Geometry check sheet. Reference: the model listing, model coordinates, mm. A direction names the side the tool comes from. Round coordinates to 2 decimals unless told otherwise and drop trailing zeros. Order: outer loops, then holes, each group sorted by start corner. A loop starts at its lowest first (then second) coordinate and runs counter-clockwise, first axis right, second up.
(1) Cross-section at B-B on x = 29. Enter the section's corners in (y, z).
(2) Set-up check for faces 1 (the face through (6.2, 3, -10)), 2 (the face through (8.6, 5.2, -14.2)), 3 (the face through (26.78, 3, -32)), 4 (the face through (3, 3, -24.66)), 5 (the face through (12, 3, -35)): record each of +Z, -Z, +X, -X, +Y, -Y from which the full face is reachable in a straight line by a thin tool's end or side.
(3) Gauge pin test, flat ends, axial feed: P1, Ø2, axis at x = 16, y = 2.5, coming from the -Z side; P2, Ø3, axis at x = 2, y = 3.5, coming from the +Z side; P3, Ø3, axis at y = 2, z = -33, coming from the -X side. Record the tip position at first contact, or that the pin passes through.
(4) Thickness scan on L1, parallel to X at y = 2, z = -32.5; L2, parallel to X at y = 3.5, z = -25; L3, parallel to Z at x = 30.5, y = 2.75. Record the ranges inside material, lowest first.
(5) Cross-section at C-C on z = -20. Enter the section's corners in (x, y).
(6) Cross-section at D-D on y = 2. Count the separate pieces of the cut face and the enclosed holes in it, and give its area (3 significant figures).
(7) Draft check along Z on faces 6 (the face through (3, 3, -4.11)), 7 (the face through (7.9, 5.71, -14.66)), 8 (the face through (0, 3, -6)). Enter one of: pulls with the +Z half, pulls with the -Z half, needs draft (parallel to the pull), parting line crosses it, or undercut.
(8) Cross-section at A-A on x = 5.5. Enter the section's corners in (y, z).
from build123d import *

# Parameters (mm, degrees)
SKETCH1_R           = 2.5
BOSS_EXTRUDE1_DEPTH = 6.2
CUT_EXTRUDE1_DEPTH  = 1


with BuildPart() as part:
    # Sketch1 → Boss-Extrude1 (new body)
    with BuildSketch(Plane(origin=(0, 0, 0), x_dir=(1, 0, 0), z_dir=(0, 1, 0))):
        Polygon((0, 24.66), (0, 20.55), (6.2, 20.55), (6.2, 16.44), (0, 16.44), (0, 12.33), (6.2, 12.33), (6.2, 8.22), (0, 8.22), (0, 4.11), (6.2, 4.11), (6.2, 0), (17, 0), (35, 0), (35, 18), (35, 28.8), (30.89, 28.8), (30.89, 35), (26.78, 35), (26.78, 28.8), (22.67, 28.8), (22.67, 35), (18.56, 35), (18.56, 28.8), (14.45, 28.8), (14.45, 35), (10.34, 35), (10.34, 28.8), (6.2, 28.8), (6.2, 24.66), align=None)
        with Locations((10.006, 25)):
            Circle(SKETCH1_R, mode=Mode.SUBTRACT)
        with Locations((30.02235364, 4.980572344)):
            Circle(SKETCH1_R, mode=Mode.SUBTRACT)
    extrude(amount=BOSS_EXTRUDE1_DEPTH)

    # Sketch2 → Cut-Extrude1 (cut)
    with BuildSketch(Plane(origin=(0, 6.2, 0), x_dir=(1, 0, 0), z_dir=(0, 1, 0))):
        with BuildLine():
            Line((9.367624272, 15.46006193), (9.367624272, 15.134420905))
            Line((9.367624272, 15.134420905), (8.28766634, 15.134420905))
            Line((8.28766634, 15.134420905), (8.116577598, 14.299329759))
            add(Edge.make_bspline(
                [(8.116577598, 14.299329759), (8.150192569, 14.308610077), (8.215316261, 14.326589225), (8.311436992, 14.346551603), (8.40268849, 14.358585256), (8.461902576, 14.360228373), (8.490555963, 14.361023469)],
                knots=[0, 0, 0, 0, 0.000104595, 0.000202637, 0.000294305, 0.000380252, 0.000380252, 0.000380252, 0.000380252], degree=3))
            add(Edge.make_bspline(
                [(8.490555963, 14.361023469), (8.526010498, 14.360256084), (8.595722973, 14.358747215), (8.697721161, 14.344258466), (8.795087428, 14.321452972), (8.88761815, 14.289593641), (8.975484506, 14.248854097), (9.05787808, 14.197963437), (9.136035615, 14.138515344), (9.208554968, 14.070166655), (9.274344876, 13.994944902), (9.332189738, 13.914065976), (9.381322945, 13.828315883), (9.420838773, 13.736875331), (9.452393133, 13.640755241), (9.4733953, 13.538944256), (9.487380458, 13.432402033), (9.488942908, 13.359554316), (9.489739657, 13.322406682)],
                knots=[0, 0, 0, 0, 0.000106308, 0.000209029, 0.000308378, 0.000405929, 0.000502102, 0.000598312, 0.00069588, 0.000796219, 0.000896736, 0.000995218, 0.001094066, 0.001192613, 0.001293582, 0.001396995, 0.001504047, 0.001615439, 0.001615439, 0.001615439, 0.001615439], degree=3))
            add(Edge.make_bspline(
                [(9.489739657, 13.322406682), (9.489136339, 13.296532954), (9.487937855, 13.245135158), (9.481843137, 13.168804347), (9.470108594, 13.094089491), (9.454353587, 13.020980679), (9.433904394, 12.94961632), (9.409149323, 12.879792148), (9.378854356, 12.811942755), (9.345624465, 12.745426146), (9.308208017, 12.681746072), (9.266680371, 12.622193063), (9.222805961, 12.56587375), (9.17559699, 12.51339215), (9.124614659, 12.465093126), (9.070476403, 12.420690042), (9.013614223, 12.379431978), (8.953148396, 12.342993687), (8.890426286, 12.309463005), (8.824542118, 12.281955225), (8.756995625, 12.257362103), (8.686814631, 12.237759175), (8.614158101, 12.222398929), (8.538906269, 12.211966241), (8.461453804, 12.204367616), (8.4089529, 12.203891949), (8.382432966, 12.203651674)],
                knots=[0, 0, 0, 0, 7.7636e-05, 0.000154223, 0.000229512, 0.000304362, 0.000378447, 0.000452077, 0.000526407, 0.000601214, 0.00067506, 0.000747747, 0.00081887, 0.000889121, 0.000959302, 0.001029336, 0.001099058, 0.00116985, 0.001240974, 0.00131221, 0.00138383, 0.001456517, 0.001530612, 0.001606437, 0.001684346, 0.001763871, 0.001763871, 0.001763871, 0.001763871], degree=3))
            add(Edge.make_bspline(
                [(8.382432966, 12.203651674), (8.350797102, 12.204278363), (8.288557277, 12.205511299), (8.197370763, 12.218409496), (8.109636799, 12.236882477), (8.026061636, 12.264673951), (7.945896275, 12.299496711), (7.870219953, 12.343507809), (7.797098999, 12.393381711), (7.729505937, 12.452237459), (7.666771462, 12.516568114), (7.610613415, 12.586379688), (7.560599385, 12.660519968), (7.517530286, 12.739349008), (7.480792795, 12.822659675), (7.451932056, 12.910764112), (7.428638119, 13.003201972), (7.418783445, 13.066841228), (7.413778118, 13.099164495)],
                knots=[0, 0, 0, 0, 9.4843e-05, 0.000186593, 0.000275792, 0.000363484, 0.000450342, 0.000537514, 0.000625728, 0.000715478, 0.000805885, 0.000894984, 0.00098389, 0.001073836, 0.001164117, 0.001256635, 0.001351658, 0.001449737, 0.001449737, 0.001449737, 0.001449737], degree=3))
            Line((7.413778118, 13.099164495), (7.698714016, 13.099164495))
            add(Edge.make_bspline(
                [(7.698714016, 13.099164495), (7.705724921, 13.068887284), (7.719200271, 13.010692804), (7.748778343, 12.928930802), (7.784942388, 12.856069792), (7.827944904, 12.791145956), (7.87924386, 12.73453208), (7.93778127, 12.684079459), (8.003410991, 12.638563449), (8.076339135, 12.600624224), (8.153276714, 12.56826757), (8.233801254, 12.546721389), (8.315720197, 12.531571293), (8.371127004, 12.530054768), (8.398969424, 12.5292927)],
                knots=[0, 0, 0, 0, 9.3172e-05, 0.000179081, 0.000260145, 0.000336703, 0.000411917, 0.000488562, 0.000568128, 0.000650923, 0.00073478, 0.000817953, 0.000900557, 0.000983994, 0.000983994, 0.000983994, 0.000983994], degree=3))
            add(Edge.make_bspline(
                [(8.398969424, 12.5292927), (8.426146013, 12.530037262), (8.479656939, 12.531503313), (8.558407269, 12.542787274), (8.634437519, 12.560165928), (8.706997478, 12.586173582), (8.777356875, 12.617782719), (8.843735938, 12.658345681), (8.908054976, 12.705027269), (8.968314783, 12.758509355), (9.023504855, 12.817446149), (9.072269336, 12.880472071), (9.112888394, 12.947706638), (9.147118621, 13.017985856), (9.173111256, 13.092079975), (9.191654146, 13.169641756), (9.202542635, 13.250862773), (9.204040492, 13.306261362), (9.204803759, 13.334491017)],
                knots=[0, 0, 0, 0, 8.15e-05, 0.000160473, 0.000238226, 0.000315066, 0.000391338, 0.000469218, 0.000547964, 0.000629516, 0.000710512, 0.000789892, 0.000868102, 0.000945761, 0.001024012, 0.00110315, 0.001184644, 0.001269321, 0.001269321, 0.001269321, 0.001269321], degree=3))
            add(Edge.make_bspline(
                [(9.204803759, 13.334491017), (9.204206424, 13.359959735), (9.203037226, 13.409811125), (9.193484495, 13.482744691), (9.176868384, 13.551753808), (9.153805293, 13.61717172), (9.124523168, 13.679060129), (9.088739728, 13.737482905), (9.045783431, 13.791670025), (8.996714361, 13.841646841), (8.942958852, 13.887770406), (8.883592028, 13.927089685), (8.819856238, 13.960167667), (8.752519387, 13.988713637), (8.6799798, 14.009215742), (8.603673998, 14.024608038), (8.522777984, 14.033511974), (8.46746886, 14.034747402), (8.439038535, 14.035382443)],
                knots=[0, 0, 0, 0, 7.6388e-05, 0.000149519, 0.000220172, 0.000288967, 0.000357247, 0.000425206, 0.000494043, 0.000564207, 0.000635056, 0.000706145, 0.000777268, 0.000850264, 0.000925136, 0.001002969, 0.001083601, 0.001168886, 0.001168886, 0.001168886, 0.001168886], degree=3))
            add(Edge.make_bspline(
                [(8.439038535, 14.035382443), (8.414428721, 14.034855764), (8.363615699, 14.033768305), (8.28567142, 14.025761412), (8.203763929, 14.012844338), (8.118207208, 13.995076813), (8.028744318, 13.971825765), (7.935564055, 13.943963325), (7.838470499, 13.910651226), (7.77304942, 13.885494147), (7.739419144, 13.87256193)],
                knots=[0, 0, 0, 0, 7.3822e-05, 0.000152423, 0.000234822, 0.000322511, 0.00041445, 0.000512043, 0.000614219, 0.000722306, 0.000722306, 0.000722306, 0.000722306], degree=3))
            Line((7.739419144, 13.87256193), (8.06506017, 15.46006193))
            Line((8.06506017, 15.46006193), (9.367624272, 15.46006193))
        make_face()
        Polygon((11.548528719, 15.541472187), (11.606406324, 15.541472187), (11.606406324, 13.343395264), (11.972752477, 13.343395264), (11.972752477, 13.017754238), (11.606406324, 13.017754238), (11.606406324, 12.28506193), (11.321470426, 12.28506193), (11.321470426, 13.017754238), (9.815380682, 13.017754238), align=None)
        Polygon((11.321470426, 13.343395264), (11.321470426, 14.722281482), (10.375076195, 13.343395264), align=None, mode=Mode.SUBTRACT)
    extrude(amount=-CUT_EXTRUDE1_DEPTH, mode=Mode.SUBTRACT)


solid = part.part
Found:
1. outline: (0, -35) - (6.2, -35) - (6.2, -7.26) - (0, -7.26) - close; (0, -2.7) - (6.2, -2.7) - (6.2, 0) - (0, 0) - close
2. face 1: -X, +Y, -Y
2. face 2: +Y
2. face 3: -Z, +Y, -Y
2. face 4: -Z, -X, +Y, -Y
2. face 5: -Z, +X, -X, +Y, -Y
3. P1: stops at z = -28.8
3. P2: stops at z = -4.11
3. P3: stops at x = 10.34
4. L1: x = 10.34 to 14.45, 18.56 to 22.67, 26.78 to 30.89
4. L2: x = 6.2 to 7.51, 12.51 to 35
4. L3: z = -35 to -7.43, -2.53 to 0
5. outline: (6.2, 0) - (35, 0) - (35, 6.2) - (6.2, 6.2) - close
6. separate pieces: 1
6. enclosed holes: 2
6. area: 943 mm2
7. face 6: pulls with the +Z half
7. face 7: undercut
7. face 8: needs draft
8. outline: (0, -24.66) - (6.2, -24.66) - (6.2, -20.55) - (0, -20.55) - close; (0, -16.44) - (6.2, -16.44) - (6.2, -12.33) - (0, -12.33) - close; (0, -8.22) - (6.2, -8.22) - (6.2, -4.11) - (0, -4.11) - close
